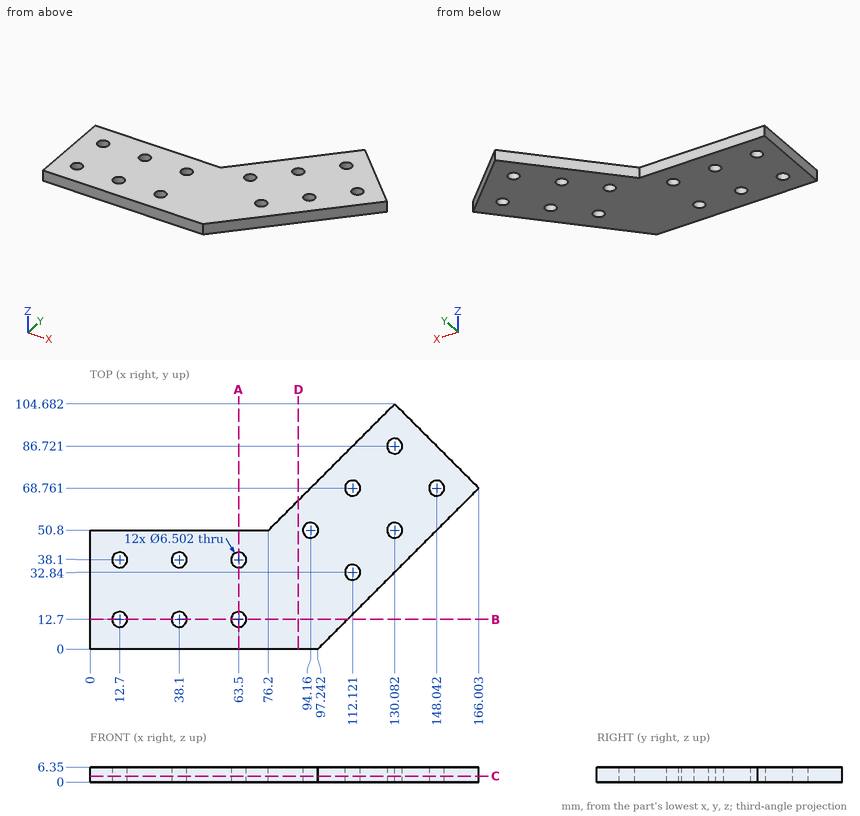
The drawing under review shows one solid part. Ordinate dimensions are in mm from its lowest x, y, z. Round coordinates to 2 decimals unless told otherwise and drop trailing zeros. Loops run counter-clockwise (first coordinate to the right, second up) from the corner with the lowest first, then second, coordinate; pieces in that order, holes last. Notation, with made-up numbers: (-24, 60) -> (-4, 60) arc R4 cw to (-4, 65) -> close; hole circle Ø6 at (55, -8). An arc over 180 degrees is marked (long way). Answer in a Markdown table with one row per item.
1) Consider section C-C, the plane z = 2.5. Count the separate pieces of the cut face and the enclosed holes in it, plus the area to 3 significant figures.
Taken from the geometry:
| item | result |
|---|---|
| separate pieces | 1 |
| enclosed holes | 12 |
| area | 8,410 mm² |
2) Consider section A-A, the plane x = 63.5. Write out the cut boundary in (y, z).
Taken from the geometry:
| item | result |
|---|---|
| outline | (0, 0) -> (9.45, 0) -> (9.45, 6.35) -> (0, 6.35) -> close; (15.95, 0) -> (34.85, 0) -> (34.85, 6.35) -> (15.95, 6.35) -> close; (41.35, 0) -> (50.8, 0) -> (50.8, 6.35) -> (41.35, 6.35) -> close |
3) Consider section B-B, the plane y = 12.7. Write out the cut boundary in (x, z), plus the area to 3 significant figures.
Taken from the geometry:
| item | result |
|---|---|
| outline | (0, 0) -> (9.45, 0) -> (9.45, 6.35) -> (0, 6.35) -> close; (15.95, 0) -> (34.85, 0) -> (34.85, 6.35) -> (15.95, 6.35) -> close; (41.35, 0) -> (60.25, 0) -> (60.25, 6.35) -> (41.35, 6.35) -> close; (66.75, 0) -> (109.94, 0) -> (109.94, 6.35) -> (66.75, 6.35) -> close |
| area | 574 mm² |
4) Consider section D-D, the plane x = 89. Write out the cut boundary in (y, z), plus the area to 3 significant figures.
Taken from the geometry:
| item | result |
|---|---|
| outline | (0, 0) -> (63.6, 0) -> (63.6, 6.35) -> (0, 6.35) -> close |
| area | 404 mm² |
5) Wall thickness on line 1 along Y through (x, z) = (63.5, 3.25); line 2 along Y through (x, z) = (47, 1); line 3 along Y through (x, z) = (61, 5.5): over which ranges is each line inside the solid? List them lowest first.
Taken from the geometry:
| item | result |
|---|---|
| line 1 | y = 0 to 9.45, 15.95 to 34.85, 41.35 to 50.8 |
| line 2 | y = 0 to 50.8 |
| line 3 | y = 0 to 10.62, 14.78 to 36.02, 40.18 to 50.8 |
